Geometry: final body of the model. Coordinates: model frame, mm. Face numbers are marked on the shaded views. A direction names the side the tool comes from. Coordinates: 2 decimals unless noted, no trailing zeros. Order: outer loops, then holes, each group sorted by start corner. A loop starts at its lowest first (then second) coordinate and runs counter-clockwise, first axis right, second up. Notation, with made-up numbers: (47.25, 30.25) -> (93.25, 30.25) arc R13 cw to (93.25, 34.25) -> close; hole circle Ø10 at (26.5, -1.75). An arc over 180 degrees is marked (long way). Use one line per item in the form item = value.
Autodesk Fusion 360 part; units mm, degrees
sketch "Sketch1" plane through (0, 0, 0) normal (0, 0, 1) x (1, 0, 0)
  circle A0 centre (0, 0) radius 3.75
  circle A1 centre (0, 0) radius 1.25
  circle A2 centre (0, 0) radius 4.75
  line L0 (0, 0) -> (0, -4.75)
  line L1 (0, -4.75) -> (2.5, -4.75)
  line L2 (0, -4.75) -> (-2.5, -4.75)
  line L3 (2.5, -4.75) -> (2.5, -2.7951)
  line L4 (-2.5, -4.75) -> (-2.5, -2.7951)
  line L5 (2.5, -4.75) -> (4.75, -4.75)
  line L6 (4.75, -4.75) -> (4.75, 0)
  line L7 (-4.75, 0) -> (-4.75, -4.75)
  line L8 (-4.75, -4.75) -> (-2.5, -4.75)
  dimension "d1" = 7.5
  dimension "d2" = 2.5
  dimension "d3" = 9.5
  dimension "d4" = 2.5
  dimension "d5" = 2.5
  dimension "d10" = 2.25
extrude "Extrude1" add sketch "Sketch1" along normal blind 5 contours A0 | A0 A2 L0 L4 | A0 A2 L0 L3 | A2 L2 L4 | A2 L1 L3
extrude "Extrude2" add sketch "Sketch1" along normal blind 2 contours A1
extrude "Extrude3" add sketch "Sketch1" against normal blind 1.25 contours A1 | A0 | A0 A2 L3 L4 | A0 A2 L0 L4 | A0 A2 L0 L3 | A2 L4 L7 L8 | A2 L2 L4 | A2 L1 L3 | A2 L3 L5 L6
extrude "Extrude4" add 1 faces at (-0.9543, -2.5804, 5) along direction (0, 0, 1) blind 6.444
extrude "Extrude5" [suppressed]
extrude "Extrude6" [suppressed]
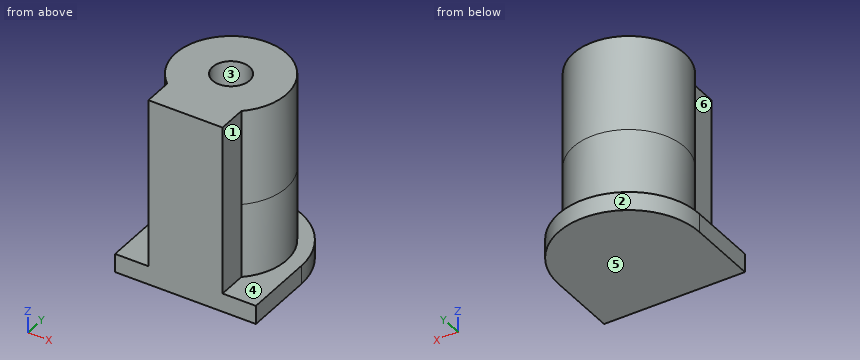
1) Pull-direction query (Y, two-part tool) for the marked faces 1, 2 and 3; classes: released by +Y, released by -Y, zero draft, split by the parting line, or undercut.
Results found:
face_1 = zero draft
face_2 = released by +Y
face_3 = undercut
2) Section A-A, the plane x = 0. Output: boundary loops of the cut face in (y, z), and give its area (3 significant figures).
Results found:
outline = (-4.75, -1.25) -> (4.75, -1.25) -> (4.75, 0) -> (3.75, 0) -> (3.75, 11.44) -> (1.25, 11.44) -> (1.25, 2) -> (-1.25, 2) -> (-1.25, 11.44) -> (-4.75, 11.44) -> close
area = 85.5 mm2
3) Material intervals for probe 1 along X at (y, z) = (0, 5.5); probe 2 along Y at (x, z) = (0, 3.5); probe 3 along Y at (x, z) = (0.75, 3), sorted ascending. Write a range as from..to.
Results found:
probe_1 = -3.75..-1.25, 1.25..3.75
probe_2 = -4.75..-1.25, 1.25..3.75
probe_3 = -4.75..-1, 1..3.67
4) Section D-D, the plane z = 0.5. Output: boundary loops of the cut face in (x, y), and give its area (3 significant figures).
Results found:
outline = (-2.5, -4.75) -> (2.5, -4.75) -> (2.5, -2.8) arc R3.75 ccw (long way) to (-2.5, -2.8) -> close
area = 50.7 mm2
5) Access query for the marked faces 4, 5 and 6. Directions: +Z, -Z, +X, -X, +Y, -Y. A direction counts if a zero-diameter tool reaches every point of the face in a straight line with its end or side. Return the directions, or none.
Results found:
face_4 = +Z
face_5 = -Z, +X, -X, +Y, -Y
face_6 = +Z, -X, -Y
6) Section C-C, the plane y = -3. Output: boundary loops of the cut face in (x, z).
Results found:
outline = (-4.75, -1.25) -> (4.75, -1.25) -> (4.75, 0) -> (2.5, 0) -> (2.5, 11.44) -> (-2.5, 11.44) -> (-2.5, 0) -> (-4.75, 0) -> close
7) Contact query for flat-ended pins moving along their axis: P1, Ø1, axis at y = -3.5, z = 5.5, coming from the -X side; P2, Ø5, axis at y = -2, z = 9.5, coming from the +X side; P3, Ø2, axis at y = -3.5, z = 5.5, coming from the +X side. Output: stop coordinate, or through.
Results found:
P1 = -2.5
P2 = 3.75
P3 = 2.8
8) Section B-B, the plane z = 8.5. Output: boundary loops of the cut face in (x, y), and give its area (3 significant figures).
Results found:
outline = (-2.5, -4.75) -> (2.5, -4.75) -> (2.5, -2.8) arc R3.75 ccw (long way) to (-2.5, -2.8) -> close; hole circle Ø2.5 at (0, 0)
area = 45.8 mm2
